```python
from build123d import *

# Parameters (mm, degrees)
EXTRUDE_1_DEPTH     = 3
SKETCH_2_R          = 1
CUT_EXTRUDE_1_DEPTH = 3
EXTRUDE_2_DEPTH     = 3
CHAMFER_1_SIZE      = 0.25
EXTRUDE_START       = 3
SKETCH_4_R          = 2.5
SKETCH_4_R_2        = 1
EXTRUDE_3_DEPTH     = 3
CHAMFER_3_SIZE      = 0.25


with BuildPart() as part:
    # 草图1 → 凸台-拉伸1 (new body)
    with BuildSketch(Plane(origin=(0, 0, 0), x_dir=(1, 0, 0), z_dir=(0, 1, 0))):
        with BuildLine():
            Line((2, 1.5), (18, 1.5))
            ThreePointArc((18, 1.5), (22.5, 0), (18, -1.5))
            Line((18, -1.5), (2, -1.5))
            ThreePointArc((2, -1.5), (-2.5, 0), (2, 1.5))
        make_face()
    extrude(amount=EXTRUDE_1_DEPTH)

    # 草图2 → 切除-拉伸1 (cut)
    with BuildSketch(Plane(origin=(0, 0, 0), x_dir=(1, 0, 0), z_dir=(0, 1, 0))):
        with Locations(Location((0, 0, 0), (0, 0, 270))):
            Circle(SKETCH_2_R)
        with Locations(Location((20, 0, 0), (0, 0, 270))):
            Circle(SKETCH_2_R)
    extrude(amount=CUT_EXTRUDE_1_DEPTH, mode=Mode.SUBTRACT)

    # 草图3 → 凸台-拉伸2 (add)
    with BuildSketch(Plane(origin=(0, 0, 0), x_dir=(1, 0, 0), z_dir=(0, 1, 0))):
        with BuildLine():
            Line((4.5, 1.5), (0.578145188, 2.432231104))
            ThreePointArc((0.578145188, 2.432231104), (1.370755945, 2.090700395), (2, 1.5))
            Line((2, 1.5), (4.5, 1.5))
        make_face()
        with BuildLine():
            Line((4.5, -1.5), (0.578145188, -2.432231104))
            ThreePointArc((0.578145188, -2.432231104), (1.370755945, -2.090700395), (2, -1.5))
            Line((2, -1.5), (4.5, -1.5))
        make_face()
        with BuildLine():
            Line((18, 1.5), (15.5, 1.5))
            Line((15.5, 1.5), (19.421854812, 2.432231104))
            ThreePointArc((19.421854812, 2.432231104), (18.629244055, 2.090700395), (18, 1.5))
        make_face()
        with BuildLine():
            Line((15.5, -1.5), (19.421854812, -2.432231104))
            ThreePointArc((19.421854812, -2.432231104), (18.629244055, -2.090700395), (18, -1.5))
            Line((18, -1.5), (15.5, -1.5))
        make_face()
    extrude(amount=EXTRUDE_2_DEPTH)

    # 倒角1
    chamfer_1_edges = [part.edges().sort_by_distance(p)[0] for p in [
        (0, 0, -1),
        (20, 0, -1),
        (-2.5, 0, 0),
        (2.539072594, 0, -1.966115552),
        (10, 0, 1.5),
        (2.539072594, 0, 1.966115552),
        (22.5, 0, 0),
        (17.460927406, 0, 1.966115552),
        (10, 0, -1.5),
        (17.460927406, 0, -1.966115552),
    ]]
    chamfer(chamfer_1_edges, length=CHAMFER_1_SIZE)

    # 草图4 → 凸台-拉伸3 (add)
    with BuildSketch(Plane(origin=(0, 0, 0), x_dir=(1, 0, 0), z_dir=(0, 1, 0)).offset(EXTRUDE_START)):
        with Locations(Location((20, 0, 0), (0, 0, 103.371151196))):
            Circle(SKETCH_4_R)
        with Locations(Location((20, 0, 0), (0, 0, 270))):
            Circle(SKETCH_4_R_2, mode=Mode.SUBTRACT)
    extrude(amount=EXTRUDE_3_DEPTH)

    # 倒角3
    chamfer_3_edges = [part.edges().sort_by_distance(p)[0] for p in [
        (0, 3, -1),
        (-2.5, 3, 0),
        (2.539072594, 3, -1.966115552),
        (10, 3, 1.5),
        (2.539072594, 3, 1.966115552),
        (10, 3, -1.5),
        (20.578145188, 6, 2.432231104),
        (20, 6, -1),
    ]]
    chamfer(chamfer_3_edges, length=CHAMFER_3_SIZE)


solid = part.part
```
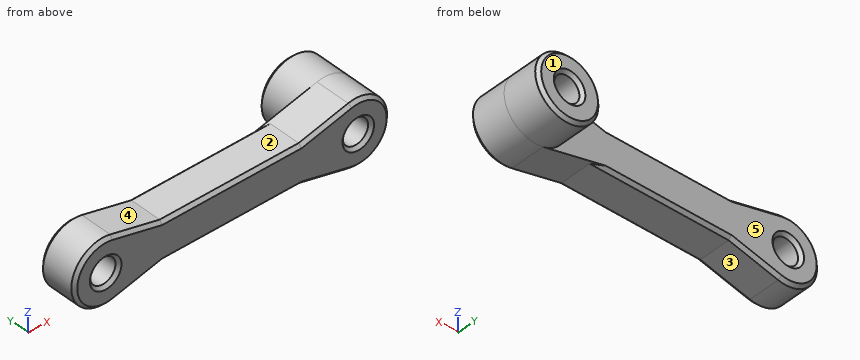
The model under review builds one solid part; all positions refer to its coordinate system, in mm. Face numbers are marked on the shaded views. A direction names the side the tool comes from. Give positions to 0.01 mm unless a question says otherwise; leave off trailing zeros. Write each loop counter-clockwise with the first axis right and the second up, starting at its lowest first coordinate (ties: lowest second). Pieces come first, ordered by that corner, then holes. Notation, with made-up numbers: M -25.75,87.25 L -19.75,87.25 A8 ccw -19.75,94.25 Z; hole C 1.5,62 d6. An arc over 180 degrees is marked long. Write each question's results on one line, items separated by ' | '. Start each with the question number.
1. Mouldability with a two-part tool opening along X and no side actions: class the marked faces 4 and 5 as released by +X, released by -X, zero draft, split by the parting line, or undercut.
2. For probe 1 along X at (y, z) = (1.45, 0); probe 2 along X at (y, z) = (1.6, -0.9); probe 3 along Y at (x, z) = (9.75, 0.3), list the stretches that pass through material, from the lowest coordinate up. Write a range as [from, to].
3. We need section B-B (z = 0). Write out the cut boundary in (x, y).
4. For the marked faces 1, 2 and 3, list the 3-axis set-ups (+Z, -Z, +X, -X, +Y, -Y) from which the entire face can be reached by the end or side of a thin tool; tool diameter is ignored.
5. We need section A-A (y = 1.9). Write out the cut boundary in (x, z), and give its area (3 significant figures).
6. Insertion check: pin 1 Ø1 at (y, z) = (1, 0.5) entering from +X; pin 2 Ø0.8 at (x, y) = (11.5, 2) entering from -Z; pin 3 Ø2 at (x, y) = (10.5, 2) entering from +Z; pin 4 Ø1 at (y, z) = (1.5, 1.5) entering from +X. Each pin has a flat end and moves straight along its axis. Give the tip position at first contact, or say it passes through.
7. We need section D-D (x = 12.75). Write out the cut boundary in (y, z), and give its area (4 significant figures).
8. We need section C-C (x = 20). Write out the cut boundary in (y, z), and give its area (4 significant figures).
Results found:
1) face 4: undercut | face 5: zero draft
2) probe 1: x = [-2.5, -1], [1, 19], [21, 22.5] | probe 2: x = [-2.33, -0.44], [0.44, 19.56], [20.44, 22.33] | probe 3: y = [0, 3]
3) outline: M -2.5,0.25 L -2.25,0 L -1.25,0 L -1,0.25 L -1,2.75 L -1.25,3 L -2.25,3 L -2.5,2.75 Z; M 1,0.25 L 1.25,0 L 18.75,0 L 19,0.25 L 19,5.75 L 18.75,6 L 17.75,6 L 17.5,5.75 L 17.5,3 L 1.25,3 L 1,2.75 Z; M 21,0.25 L 21.25,0 L 22.25,0 L 22.5,0.25 L 22.5,5.75 L 22.25,6 L 21.25,6 L 21,5.75 Z
4) face 1: +Z, -Z, +X, -X, +Y | face 2: +Z, +Y, -Y | face 3: -Z, +Y, -Y
5) outline: M 0.58,-2.43 L 4.5,-1.5 L 15.5,-1.5 L 19.42,-2.43 A2.5 ccw long 19.42,2.43 L 15.5,1.5 L 4.5,1.5 L 0.58,2.43 A2.5 ccw long Z; hole C 0,0 d2; hole C 20,0 d2 | area: 82.9 mm^2
6) pin 1: stops at x = 22.5 | pin 2: stops at z = -1.5 | pin 3: stops at z = 1.5 | pin 4: stops at x = 22.29
7) outline: M 0,-1.25 L 0.25,-1.5 L 2.75,-1.5 L 3,-1.25 L 3,1.25 L 2.75,1.5 L 0.25,1.5 L 0,1.25 Z | area: 8.875 mm^2
8) outline: M 0,-2.25 L 0.25,-2.5 L 5.75,-2.5 L 6,-2.25 L 6,-1.25 L 5.75,-1 L 0.25,-1 L 0,-1.25 Z; M 0,1.25 L 0.25,1 L 5.75,1 L 6,1.25 L 6,2.25 L 5.75,2.5 L 0.25,2.5 L 0,2.25 Z | area: 17.75 mm^2
